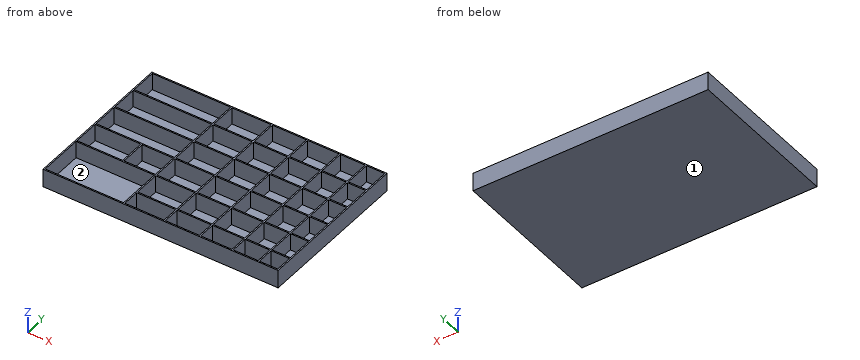
from build123d import *

# Parameters (mm, degrees)
F0_W     = 180
F0_H     = 120
F1_DEPTH = 1
F2_W     = 180
F2_H     = 120
F2_W_2   = 60
F2_H_2   = 34
F2_W_3   = 30
F2_H_3   = 13
F2_H_4   = 20
F2_W_4   = 35
F2_W_5   = 24
F2_W_6   = 26
F2_W_7   = 19
F2_W_8   = 14
F3_DEPTH = 14


with BuildPart() as f1:
    # F0 (on Top) → F1 (new body)
    with BuildSketch(Plane.XY):
        with Locations((-23.763961, -4.79302)):
            Rectangle(F0_W, F0_H)
    extrude(amount=F1_DEPTH)

    # F2 (on Top) → F3 (join)
    with BuildSketch(Plane.XY):
        with Locations((-23.763961, -4.79302)):
            Rectangle(F2_W, F2_H)
        with Locations((-82.763961, -46.79302)):
            Rectangle(F2_W_2, F2_H_2, mode=Mode.SUBTRACT)
        with Locations((-36.763961, -57.29302)):
            Rectangle(F2_W_3, F2_H_3, mode=Mode.SUBTRACT)
        with Locations((-36.763961, -39.79302)):
            Rectangle(F2_W_3, F2_H_4, mode=Mode.SUBTRACT)
        with Locations((-95.263961, -18.79302)):
            Rectangle(F2_W_4, F2_H_4, mode=Mode.SUBTRACT)
        with Locations((-64.763961, -18.79302)):
            Rectangle(F2_W_5, F2_H_4, mode=Mode.SUBTRACT)
        with Locations((-36.763961, -18.79302)):
            Rectangle(F2_W_3, F2_H_4, mode=Mode.SUBTRACT)
        with Locations((-7.763961, -57.29302)):
            Rectangle(F2_W_6, F2_H_3, mode=Mode.SUBTRACT)
        with Locations((18.236039, -57.29302)):
            Rectangle(F2_W_5, F2_H_3, mode=Mode.SUBTRACT)
        with Locations((-7.763961, -39.79302)):
            Rectangle(F2_W_6, F2_H_4, mode=Mode.SUBTRACT)
        with Locations((18.236039, -39.79302)):
            Rectangle(F2_W_5, F2_H_4, mode=Mode.SUBTRACT)
        with Locations((40.736039, -57.29302)):
            Rectangle(F2_W_7, F2_H_3, mode=Mode.SUBTRACT)
        with Locations((58.236039, -57.29302)):
            Rectangle(F2_W_8, F2_H_3, mode=Mode.SUBTRACT)
        with Locations((40.736039, -39.79302)):
            Rectangle(F2_W_7, F2_H_4, mode=Mode.SUBTRACT)
        with Locations((58.236039, -39.79302)):
            Rectangle(F2_W_8, F2_H_4, mode=Mode.SUBTRACT)
        with Locations((-7.763961, -18.79302)):
            Rectangle(F2_W_6, F2_H_4, mode=Mode.SUBTRACT)
        with Locations((18.236039, -18.79302)):
            Rectangle(F2_W_5, F2_H_4, mode=Mode.SUBTRACT)
        with Locations((40.736039, -18.79302)):
            Rectangle(F2_W_7, F2_H_4, mode=Mode.SUBTRACT)
        with Locations((58.236039, -18.79302)):
            Rectangle(F2_W_8, F2_H_4, mode=Mode.SUBTRACT)
        with Locations((-82.763961, 2.20698)):
            Rectangle(F2_W_2, F2_H_4, mode=Mode.SUBTRACT)
        with Locations((-82.763961, 23.20698)):
            Rectangle(F2_W_2, F2_H_4, mode=Mode.SUBTRACT)
        with Locations((-36.763961, 2.20698)):
            Rectangle(F2_W_3, F2_H_4, mode=Mode.SUBTRACT)
        with Locations((-36.763961, 23.20698)):
            Rectangle(F2_W_3, F2_H_4, mode=Mode.SUBTRACT)
        with Locations((-82.763961, 44.20698)):
            Rectangle(F2_W_2, F2_H_4, mode=Mode.SUBTRACT)
        with Locations((-36.763961, 44.20698)):
            Rectangle(F2_W_3, F2_H_4, mode=Mode.SUBTRACT)
        with Locations((-7.763961, 2.20698)):
            Rectangle(F2_W_6, F2_H_4, mode=Mode.SUBTRACT)
        with Locations((18.236039, 2.20698)):
            Rectangle(F2_W_5, F2_H_4, mode=Mode.SUBTRACT)
        with Locations((-7.763961, 23.20698)):
            Rectangle(F2_W_6, F2_H_4, mode=Mode.SUBTRACT)
        with Locations((18.236039, 23.20698)):
            Rectangle(F2_W_5, F2_H_4, mode=Mode.SUBTRACT)
        with Locations((40.736039, 2.20698)):
            Rectangle(F2_W_7, F2_H_4, mode=Mode.SUBTRACT)
        with Locations((58.236039, 2.20698)):
            Rectangle(F2_W_8, F2_H_4, mode=Mode.SUBTRACT)
        with Locations((40.736039, 23.20698)):
            Rectangle(F2_W_7, F2_H_4, mode=Mode.SUBTRACT)
        with Locations((58.236039, 23.20698)):
            Rectangle(F2_W_8, F2_H_4, mode=Mode.SUBTRACT)
        with Locations((-7.763961, 44.20698)):
            Rectangle(F2_W_6, F2_H_4, mode=Mode.SUBTRACT)
        with Locations((18.236039, 44.20698)):
            Rectangle(F2_W_5, F2_H_4, mode=Mode.SUBTRACT)
        with Locations((40.736039, 44.20698)):
            Rectangle(F2_W_7, F2_H_4, mode=Mode.SUBTRACT)
        with Locations((58.236039, 44.20698)):
            Rectangle(F2_W_8, F2_H_4, mode=Mode.SUBTRACT)
    extrude(amount=F3_DEPTH)


solid = f1.part
For this review, take the finished solid that the model builds, in its own axes (mm). Face numbers are marked on the shaded views. Round coordinates to 2 decimals unless told otherwise and drop trailing zeros. Loops run counter-clockwise (first coordinate to the right, second up) from the corner with the lowest first, then second, coordinate; pieces in that order, holes last. Notation, with made-up numbers: (-4.5, 89.5) - (19.5, 89.5) arc R19 cw to (19.5, 114.5) - close; hole circle Ø3 at (35.25, -31.75). An arc over 180 degrees is marked (long way). Put each result on its own line as item: value. Start each with the question number.
1. Consider section B-B on x = 25. State the section outline as (y, z) points.
2. Consider section C-C on z = 2.75. State how many separate pieces and enclosed holes the cut face has, plus the area to 3 significant figures.
3. Insertion check: P1, Ø10, axis at x = -32.5, y = 3, coming from the +Z side. The pin has a flat end and moves straight along its axis. Give the tip position at first contact, or say it passes through.
4. For probe 1 along Y at (x, z) = (-92.5, 4.25); probe 2 along Z at (x, y) = (-50, 39), list the stretches that pass through material, from the lowest coordinate up. Write a range as [from, to].
5. Consider section D-D on x = -82. State the section outline as (y, z) points, plus the area to 3 significant figures.
6. Mouldability with a two-part tool opening along Y and no side actions: class the marked faces 1 and 2 as +Y half, -Y half, draft (parallel to the pull), parting line (faces both ways), or undercut.
7. Consider section A-A on y = -46. State the section outline as (x, z) points, plus the area to 3 significant figures.
Result sheet:
1. outline: (-64.79, 0) - (55.21, 0) - (55.21, 14) - (54.21, 14) - (54.21, 1) - (34.21, 1) - (34.21, 14) - (33.21, 14) - (33.21, 1) - (13.21, 1) - (13.21, 14) - (12.21, 14) - (12.21, 1) - (-7.79, 1) - (-7.79, 14) - (-8.79, 14) - (-8.79, 1) - (-28.79, 1) - (-28.79, 14) - (-29.79, 14) - (-29.79, 1) - (-49.79, 1) - (-49.79, 14) - (-50.79, 14) - (-50.79, 1) - (-63.79, 1) - (-63.79, 14) - (-64.79, 14) - close
2. separate pieces: 1
2. enclosed holes: 36
2. area: 2,010 mm^2
3. P1: z = 1
4. probe 1: [-64.79, -63.79], [-29.79, -28.79], [-8.79, -7.79], [12.21, 13.21], [33.21, 34.21], [54.21, 55.21]
4. probe 2: [0, 1]
5. outline: (-64.79, 0) - (55.21, 0) - (55.21, 14) - (54.21, 14) - (54.21, 1) - (34.21, 1) - (34.21, 14) - (33.21, 14) - (33.21, 1) - (13.21, 1) - (13.21, 14) - (12.21, 14) - (12.21, 1) - (-7.79, 1) - (-7.79, 14) - (-8.79, 14) - (-8.79, 1) - (-28.79, 1) - (-28.79, 14) - (-29.79, 14) - (-29.79, 1) - (-63.79, 1) - (-63.79, 14) - (-64.79, 14) - close
5. area: 198 mm^2
6. face 1: draft
6. face 2: undercut
7. outline: (-113.76, 0) - (66.24, 0) - (66.24, 14) - (65.24, 14) - (65.24, 1) - (51.24, 1) - (51.24, 14) - (50.24, 14) - (50.24, 1) - (31.24, 1) - (31.24, 14) - (30.24, 14) - (30.24, 1) - (6.24, 1) - (6.24, 14) - (5.24, 14) - (5.24, 1) - (-20.76, 1) - (-20.76, 14) - (-21.76, 14) - (-21.76, 1) - (-51.76, 1) - (-51.76, 14) - (-52.76, 14) - (-52.76, 1) - (-112.76, 1) - (-112.76, 14) - (-113.76, 14) - close
7. area: 271 mm^2
